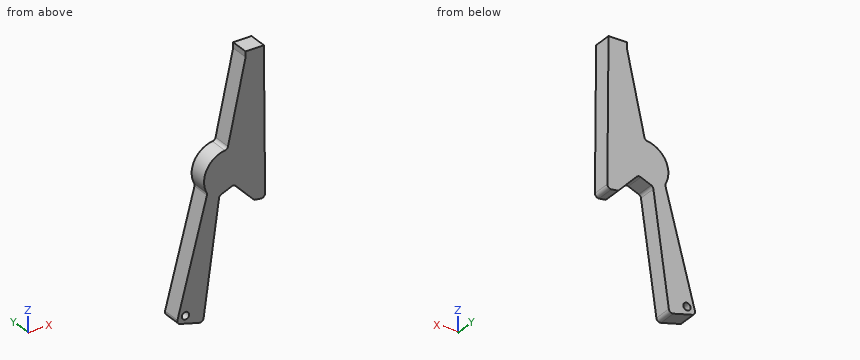
from build123d import *

# Parameters (mm, degrees)
BOSS_EXTRUDE1_DEPTH = 10
SKETCH2_R           = 2
CUT_EXTRUDE1_DEPTH  = 97.487793931
FILLET1_R           = 2


with BuildPart() as part:
    # Sketch1 → Boss-Extrude1 (new body)
    with BuildSketch(Plane(origin=(0, 0, 0), x_dir=(1, 0, 0), z_dir=(0, 1, 0))):
        with BuildLine():
            Line((23.899700969, 76.587880496), (9.410813575, 72.70559482))
            Line((9.410813575, 72.70559482), (26.234051507, 9.920416111))
            ThreePointArc((26.234051507, 9.920416111), (26.122890324, -3.007620786), (37.221477465, -9.638447153))
            Line((37.221477465, -9.638447153), (47.155900716, -54.638447153))
            Line((47.155900716, -54.638447153), (47.155900716, -57.638447153))
            Line((47.155900716, -57.638447153), (57.155900716, -57.638447153))
            Line((57.155900716, -57.638447153), (57.828980094, 22.361552847))
            Line((57.828980094, 22.361552847), (51.828980094, 21.518307839))
            Line((51.828980094, 21.518307839), (40.806779431, 9.920416111))
            Line((40.806779431, 9.920416111), (32.806779431, 13.210724097))
            Line((32.806779431, 13.210724097), (23.899700969, 76.587880496))
        make_face()
    extrude(amount=BOSS_EXTRUDE1_DEPTH)

    # Sketch2 → Cut-Extrude1 (cut, through all)
    with BuildSketch(Plane(origin=(0, 10, 0), x_dir=(1, 0, 0), z_dir=(0, 1, 0))):
        with Locations(Location((14.309793061, 69.877167695, 0), (0, 0, 270))):
            Circle(SKETCH2_R)
    extrude(amount=-CUT_EXTRUDE1_DEPTH, mode=Mode.SUBTRACT)

    # Fillet1
    fillet1_edges = [part.edges().sort_by_distance(p)[0] for p in [
        (37.221477465, 5, 9.638447153),
        (26.234051507, 5, -9.920416111),
        (9.410813575, 5, -72.70559482),
        (23.899700969, 5, -76.587880496),
        (32.806779431, 5, -13.210724097),
        (40.806779431, 5, -9.920416111),
        (57.828980094, 5, -22.361552847),
    ]]
    fillet(fillet1_edges, radius=FILLET1_R)


solid = part.part
The listing builds one solid part. Answer for the finished solid, in the listing's coordinates (mm). Round coordinates to 2 decimals unless told otherwise and drop trailing zeros. Order: outer loops, then holes, each group sorted by start corner. A loop starts at its lowest first (then second) coordinate and runs counter-clockwise, first axis right, second up. Notation, with made-up numbers: (60.5, 87.5) -> (115.5, 87.5) arc R18 cw to (115.5, 107.5) -> close; hole circle Ø2 at (76, 4). An arc over 180 degrees is marked (long way). Write each question's results on one line, items separated by ' | '. Start each with the question number.
Q1. Straight lines are drawn through the part: probe 1 along X at (y, z) = (8, -15.5); probe 2 along X at (y, z) = (9.75, -18); probe 3 along X at (y, z) = (1, 45). For each, find the intervals that lie inside material, in ascending order. Write a range as from..to.
Q2. Find section B-B (z = -46). Determine the outline of the cut face in (x, y).
Q3. Find section A-A (y = 8.5). Determine the outline of the cut face in (x, z), then the cut area to 3 significant figures.
Q4. Find section C-C (x = 18.5). Determine the outline of the cut face in (y, z).
Q5. Each of these flat-tipped pins is pushed along its axis until it touches: pin 1 (2 mm diameter, centred on x = 29.5, y = 1, fed in from +Z); pin 2 (4 mm diameter, centred on y = 2.5, z = -26, fed in from -X); pin 3 (0.9 mm diameter, centred on y = 4.5, z = 57, fed in from -X); pin 4 (3 mm diameter, centred on x = 14.31, z = -69.88, fed in from +Y). Where does it stop, or does it pass through?
Worked answers:
1) probe 1: x = 24.74..32.49, 46.11..57.77 | probe 2: x = 24.07..32.13, 48.49..57.79 | probe 3: x = 45.03..57.26
2) outline: (16.57, 0) -> (28.2, 0) -> (28.2, 10) -> (16.57, 10) -> close
3) outline: (9.93, -70.77) arc R2 ccw to (11.34, -73.22) -> (21.72, -76) arc R2 ccw to (24.21, -74.35) -> (32.65, -14.35) arc R2 cw to (33.87, -12.77) -> (39.54, -10.44) arc R2 cw to (41.75, -10.91) -> (51.83, -21.52) -> (55.53, -22.04) arc R2 ccw to (57.81, -20.04) -> (57.16, 57.64) -> (47.16, 57.64) -> (47.16, 54.64) -> (37.54, 11.09) arc R2 cw to (35.84, 9.54) arc R13 ccw to (25.88, -9.27) arc R2 cw to (26.03, -10.69) -> close; hole circle Ø4 at (14.31, -69.88) | area: 2,180 mm2
4) outline: (0, -75.14) -> (10, -75.14) -> (10, -38.78) -> (0, -38.78) -> close
5) pin 1: stops at z = 7.62 | pin 2: stops at x = 21.39 | pin 3: stops at x = 47.16 | pin 4: passes through
